The model under review builds one solid part; all positions refer to its coordinate system, in mm. A direction names the side the tool comes from. Coordinates: 2 decimals unless noted, no trailing zeros. Loops run counter-clockwise (first coordinate to the right, second up) from the corner with the lowest first, then second, coordinate; pieces in that order, holes last. Notation, with made-up numbers: (64.25, 73) -> (115.25, 73) arc R37 cw to (115.25, 110) -> close; hole circle Ø3 at (59.25, 73). An arc over 180 degrees is marked (long way). One line per question, with ' | ' between items. Start each with the question number.
from build123d import *

# Parameters (mm, degrees)
SKETCH1_W           = 26.924
SKETCH1_H           = 40.64
BOSS_EXTRUDE1_DEPTH = 19.05
SKETCH2_W           = 4.445
SKETCH2_H           = 40.64
BOSS_EXTRUDE2_DEPTH = 5.08
SKETCH3_R           = 11
CUT_EXTRUDE1_DEPTH  = 7
SKETCH4_R           = 10.16
CUT_EXTRUDE2_DEPTH  = 3.175


with BuildPart() as part:
    # Sketch1 → Boss-Extrude1 (new body)
    with BuildSketch(Plane.XY):
        Rectangle(SKETCH1_W, SKETCH1_H)
    extrude(amount=BOSS_EXTRUDE1_DEPTH)

    # Sketch2 → Boss-Extrude2 (add)
    with BuildSketch(Plane(origin=(13.462, 0, 0), x_dir=(0, 0, -1), z_dir=(1, 0, 0))):
        with Locations((-16.8275, 0)):
            Rectangle(SKETCH2_W, SKETCH2_H)
        with Locations((-2.2225, 0)):
            Rectangle(SKETCH2_W, SKETCH2_H)
    boss_extrude2 = extrude(amount=BOSS_EXTRUDE2_DEPTH)

    # Mirror1: Boss-Extrude2 across plane
    add(boss_extrude2.mirror(Plane(origin=(0, 0, 0), x_dir=(0, 0, 1), z_dir=(1, 0, 0))))

    # Sketch3 → Cut-Extrude1 (cut)
    with BuildSketch(Plane.XY.offset(19.05)):
        Circle(SKETCH3_R)
    extrude(amount=-CUT_EXTRUDE1_DEPTH, mode=Mode.SUBTRACT)

    # Sketch4 → Cut-Extrude2 (cut)
    with BuildSketch(Plane.XY.offset(12.05)):
        Circle(SKETCH4_R)
    extrude(amount=-CUT_EXTRUDE2_DEPTH, mode=Mode.SUBTRACT)


solid = part.part
1) Consider section A-A, the plane x = 0. Write out the cut boundary in (y, z) (3 decimals).
2) Consider section B-B, the plane y = 0. Write out the cut boundary in (x, z) (3 decimals), plus the area to 3 significant figures.
3) Consider section C-C, the plane x = -15.5. Write out the cut boundary in (y, z) (3 decimals).
4) Consider section D-D, the plane z = 15.5. Write out the cut boundary in (x, y), plus the area to 3 significant figures.
5) Insertion check: pin 1 Ø5.5 at (x, y) = (-17, -1) entering from -Z; pin 2 Ø13 at (x, y) = (0, 0) entering from +Z (3 decimals). Each pin has a flat end and moves straight along its axis. Give the tip position at first contact, or say it passes through.
6) Mouldability with a two-part tool opening along X and no side actions: class faces 1 (the face through (3, -10, 12.05)), 2 (the face through (18.542, 0, 17)), 3 (the face through (-2.38, -10.74, 15.6)), 4 (the face through (-18.542, 0, 17)) as +X half, -X half, draft (parallel to the pull), parting line (faces both ways), or undercut.
7) Wall thickness on L1, parallel to Z at x = 13.5, y = 0.5 (3 decimals); L2, parallel to Y at x = 0, z = 15; L3, parallel to Y at x = 0, z = 9.6: over which ranges is each line inside the solid? List them lowest first.
8) Machinability: for faces 5 (the face through (-18.542, 0, 2)), 6 (the face through (-16, 0, 4.445)), 7 (the face through (0, 0, 8.875)), 8 (the face through (16, 0, 14.605)), 9 (the face through (0, -20.32, 10)), which of the approach directions +Z, -Z, +X, -X, +Y, -Y give a long, thin tool a straight path to every point of the face, cutting with its end or side? Answer none if there is none.
Filled sheet:
1) outline: (-20.32, 0) -> (20.32, 0) -> (20.32, 19.05) -> (11, 19.05) -> (11, 12.05) -> (10.16, 12.05) -> (10.16, 8.875) -> (-10.16, 8.875) -> (-10.16, 12.05) -> (-11, 12.05) -> (-11, 19.05) -> (-20.32, 19.05) -> close
2) outline: (-18.542, 0) -> (18.542, 0) -> (18.542, 4.445) -> (13.462, 4.445) -> (13.462, 14.605) -> (18.542, 14.605) -> (18.542, 19.05) -> (11, 19.05) -> (11, 12.05) -> (10.16, 12.05) -> (10.16, 8.875) -> (-10.16, 8.875) -> (-10.16, 12.05) -> (-11, 12.05) -> (-11, 19.05) -> (-18.542, 19.05) -> (-18.542, 14.605) -> (-13.462, 14.605) -> (-13.462, 4.445) -> (-18.542, 4.445) -> close | area: 385 mm^2
3) outline: (-20.32, 0) -> (20.32, 0) -> (20.32, 4.445) -> (-20.32, 4.445) -> close; (-20.32, 14.605) -> (20.32, 14.605) -> (20.32, 19.05) -> (-20.32, 19.05) -> close
4) outline: (-18.54, -20.32) -> (18.54, -20.32) -> (18.54, 20.32) -> (-18.54, 20.32) -> close; hole circle Ø22 at (0, 0) | area: 1,130 mm^2
5) pin 1: z = 0 | pin 2: z = 8.875
6) face 1: undercut | face 2: +X half | face 3: undercut | face 4: -X half
7) L1: 0 to 4.445, 14.605 to 19.05 | L2: -20.32 to -11, 11 to 20.32 | L3: -20.32 to -10.16, 10.16 to 20.32
8) face 5: +Z, -Z, -X, +Y, -Y | face 6: -X, +Y, -Y | face 7: +Z | face 8: +X, +Y, -Y | face 9: +Z, -Z, +X, -X, -Y
